The listing builds one solid part. Answer for the finished solid, in the listing's coordinates (mm). A direction names the side the tool comes from. Round coordinates to 2 decimals unless told otherwise and drop trailing zeros. Write each loop counter-clockwise with the first axis right and the second up, starting at its lowest first coordinate (ties: lowest second). Pieces come first, ordered by that corner, then holes. Notation, with made-up numbers: M 38.5,57.25 L 44.5,57.25 A27 ccw 44.5,87.25 Z; hole C 60,8 d6. An arc over 180 degrees is marked long. Put each result on its own line as item: value. Start each with the question number.
```python
from build123d import *

# Parameters (mm, degrees)
BOSS_EXTRUDE1_DEPTH = 33
CUT_EXTRUDE1_START  = -1.5
CUT_EXTRUDE1_DEPTH  = 30


with BuildPart() as part:
    # Sketch1 → Boss-Extrude1 (new body)
    with BuildSketch(Plane.XY):
        Polygon((-37.75, -25.477481475), (-37.75, -9.477481475), (-39.75, -9.477481475), (-39.75, -23.477481475), (-63.75, -23.477481475), (-63.75, -9.477481475), (-65.75, -9.477481475), (-65.75, -25.477481475), align=None)
    extrude(amount=-BOSS_EXTRUDE1_DEPTH)

    # Sketch4 → Cut-Extrude1 (cut)
    with BuildSketch(Plane.XY.offset(CUT_EXTRUDE1_START)):
        Polygon((-65.25, -24.977481475), (-65.25, -9.477481475), (-65.75, -9.477481475), (-65.75, -25.477481475), (-37.75, -25.477481475), (-37.75, -9.477481475), (-38.25, -9.477481475), (-38.25, -24.977481475), align=None)
    extrude(amount=-CUT_EXTRUDE1_DEPTH, mode=Mode.SUBTRACT)


solid = part.part
```
Item 1: Section B-B (x = -60.5) is taken. Give the vertices of the cut face in (y, z).
Item 2: Section C-C (z = -9) is taken. Give the vertices of the cut face in (x, y), and give its area (3 significant figures).
Item 3: Section A-A (y = -23) is taken. Give the vertices of the cut face in (x, z), and give its area (3 significant figures).
Item 4: Which of the six approach directions +Z, -Z, +X, -X, +Y, -Y give full straight-line access (tool end or side, diameter ignored) to faces 1 (the flat face through (-65.25, -17, -16)), 2 (the flat face through (-52, -23.477, -16)), 3 (the flat face through (-38.25, -17, -16))?
Item 5: Flat-ended cylindrical pins translate along their axes: pin 1 (5 mm diameter, centred on y = -20.5, z = -15, fed in from +X); pin 2 (8 mm diameter, centred on y = -19, z = -11, fed in from -X); pin 3 (3 mm diameter, centred on x = -48.5, z = -21.5, fed in from -Y); pin 4 (6 mm diameter, centred on x = -41.5, z = -18, fed in from +Y). Find the tip coordinate at first contact, or state that the pin passes through.
Item 6: Consider line 1 along X through (y, z) = (-20.5, -7); line 2 along Y through (x, z) = (-58, -14.5). Determine where each line is inside the solid, lowest interval first. Write a range as [from, to].
Item 7: Determine the mould class of faces 4 (the flat face through (-51, -24, 0)), 5 (the flat face through (-51, -24, -33)), 6 (the flat face through (-39.75, -16, -16)), 7 (the flat face through (-58.04, -25.14, -1.5)) for opening direction Z: released by +Z, released by -Z, zero draft, split by the parting line, or undercut.
Output values:
1. outline: M -25.48,-33 L -23.48,-33 L -23.48,0 L -25.48,0 L -25.48,-1.5 L -24.98,-1.5 L -24.98,-31.5 L -25.48,-31.5 Z
2. outline: M -65.25,-24.98 L -38.25,-24.98 L -38.25,-9.48 L -39.75,-9.48 L -39.75,-23.48 L -63.75,-23.48 L -63.75,-9.48 L -65.25,-9.48 Z
2. area: 82.5 mm^2
3. outline: M -65.75,-33 L -63.75,-33 L -63.75,0 L -65.75,0 L -65.75,-1.5 L -65.25,-1.5 L -65.25,-31.5 L -65.75,-31.5 Z; M -39.75,-33 L -37.75,-33 L -37.75,-31.5 L -38.25,-31.5 L -38.25,-1.5 L -37.75,-1.5 L -37.75,0 L -39.75,0 Z
3. area: 102 mm^2
4. face 1: -X, +Y, -Y
4. face 2: +Z, -Z, +Y
4. face 3: +X, +Y, -Y
5. pin 1: stops at x = -38.25
5. pin 2: stops at x = -65.25
5. pin 3: stops at y = -24.98
5. pin 4: stops at y = -9.48
6. line 1: x = [-65.25, -63.75], [-39.75, -38.25]
6. line 2: y = [-24.98, -23.48]
7. face 4: released by +Z
7. face 5: released by -Z
7. face 6: zero draft
7. face 7: undercut
